Design review of the part shown in the three views and the two pictorial views. Dimensions are in mm from the part's minimum x, y and z. Round coordinates to 2 decimals unless told otherwise and drop trailing zeros. Write each loop counter-clockwise with the first axis right and the second up, starting at its lowest first coordinate (ties: lowest second). Pieces come first, ordered by that corner, then holes. Notation, with made-up numbers: (59, -34.75) - (89, -34.75) arc R32 cw to (89, 0.25) - close; hole circle Ø8 at (61.25, 5.25). An arc over 180 degrees is marked (long way). One line per item, written item: value. Start each with the question number.
Q1. Add section B-B on z = 4.3. Give the number of separate pieces and of enclosed holes in the cut face, and give its area (3 significant figures).
Q2. Clearance check with a flat-ended pin moving along its axis: pin 1 Ø2.5 at (x, y) = (65, 15) entering from -Z. State where the tip first meets the part, or that it passes through.
Q3. For probe 1 along Y at (x, z) = (55, 1.55) (3 decimals); probe 2 along X at (y, z) = (16, 0.75); probe 3 along Y at (x, z) = (64.5, 2.5), list the stretches that pass through material, from the lowest coordinate up.
Q4. Add section C-C on y = 15. Write out the cut boundary in (x, z) (3 decimals), and give its area (3 significant figures).
Q5. Add section A-A on x = 65. Write out the cut boundary in (y, z) (3 decimals).
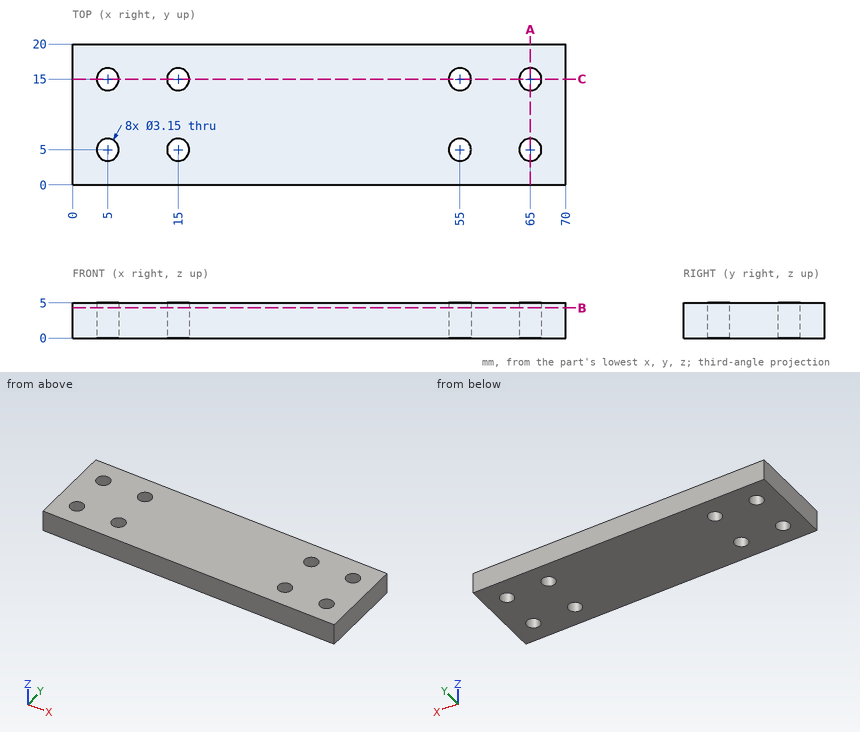
Result set:
1. separate pieces: 1
1. enclosed holes: 8
1. area: 1,340 mm^2
2. pin 1: passes through
3. probe 1: y = 0 to 3.425, 6.575 to 13.425, 16.575 to 20
3. probe 2: x = 0 to 3.78, 6.22 to 13.78, 16.22 to 53.78, 56.22 to 63.78, 66.22 to 70
3. probe 3: y = 0 to 3.51, 6.49 to 13.51, 16.49 to 20
4. outline: (0, 0) - (3.425, 0) - (3.425, 5) - (0, 5) - close; (6.575, 0) - (13.425, 0) - (13.425, 5) - (6.575, 5) - close; (16.575, 0) - (53.425, 0) - (53.425, 5) - (16.575, 5) - close; (56.575, 0) - (63.425, 0) - (63.425, 5) - (56.575, 5) - close; (66.575, 0) - (70, 0) - (70, 5) - (66.575, 5) - close
4. area: 287 mm^2
5. outline: (0, 0) - (3.425, 0) - (3.425, 5) - (0, 5) - close; (6.575, 0) - (13.425, 0) - (13.425, 5) - (6.575, 5) - close; (16.575, 0) - (20, 0) - (20, 5) - (16.575, 5) - close
